Geometry: final body of the model. Coordinates: model frame, mm. Face numbers are marked on the shaded views. Round coordinates to 2 decimals unless told otherwise and drop trailing zeros. Order: outer loops, then holes, each group sorted by start corner. A loop starts at its lowest first (then second) coordinate and runs counter-clockwise, first axis right, second up. Notation, with made-up numbers: (21.5, -37.5) - (80.5, -37.5) arc R26 cw to (80.5, -12.5) - close; hole circle Ø5 at (45.25, 53.25). An arc over 180 degrees is marked (long way). Put each result on its own line as item: value. Start each with the question number.
(1) Material intervals for L1, parallel to X at y = 9.15, z = 0; L2, parallel to X at y = 9.45, z = 18.5; L3, parallel to X at y = 8.7, z = 22, sorted ascending. Write a range as [from, to].
(2) Section C-C (z = 24). Output: boundary loops of the cut face in (x, y).
(3) Pull-direction query (Y, two-part tool) for the marked faces 1 and 2; classes: released by +Y, released by -Y, zero draft, split by the parting line, or undercut.
(4) Section B-B (y = 8.9). Output: boundary loops of the cut face in (x, z).
(5) Section D-D (z = -38). Output: boundary loops of the cut face in (x, y).
(6) Pin query (flat end, axial travel): P1, Ø0.8, axis at x = -1.5, y = 9, coming from the -Z side; P2, Ø1.5, axis at x = -32.91, z = 19, coming from the -Y side. Return the tip coordinate at first contact, or that it passes through.
(7) Section A-A (z = 0). Output: boundary loops of the cut face in (x, y).
from build123d import *

# Parameters (mm, degrees)
SKETCH_1_R      = 1.25
EXTRUDE_1_DEPTH = 1.6
FILLET_1_R      = 3


with BuildPart() as part:
    # 草图1 → 凸台-拉伸1 (new body)
    with BuildSketch(Plane(origin=(0, 8.4, 0), x_dir=(1, 0, 0), z_dir=(0, 1, 0))):
        with BuildLine():
            ThreePointArc((-42.584930161, -28.625185914), (-36.646174274, -35.915671462), (-29.47672888, -42))
            Line((-29.47672888, -42), (29.47672888, -42))
            ThreePointArc((29.47672888, -42), (36.646174274, -35.915671462), (42.584930161, -28.625185914))
            Line((42.584930161, -28.625185914), (39.709874377, -26.965271683))
            ThreePointArc((39.709874377, -26.965271683), (38.538130468, -22.25), (43.207547486, -20.90712415))
            Line((43.207547486, -20.90712415), (46.08260327, -22.567038381))
            ThreePointArc((46.08260327, -22.567038381), (44.43712591, 25.655786606), (3.497673109, 51.192224295))
            Line((3.497673109, 51.192224295), (3.497673109, 47.872395833))
            ThreePointArc((3.497673109, 47.872395833), (0, 44.5), (-3.497673109, 47.872395833))
            Line((-3.497673109, 47.872395833), (-3.497673109, 51.192224295))
            ThreePointArc((-3.497673109, 51.192224295), (-44.43712591, 25.655786606), (-46.08260327, -22.567038381))
            Line((-46.08260327, -22.567038381), (-43.207547486, -20.90712415))
            ThreePointArc((-43.207547486, -20.90712415), (-38.538130468, -22.25), (-39.709874377, -26.965271683))
            Line((-39.709874377, -26.965271683), (-42.584930161, -28.625185914))
        make_face()
        with Locations(Location((-32.908965344, -19, 0), (0, 0, 270))):
            Circle(SKETCH_1_R, mode=Mode.SUBTRACT)
        with Locations(Location((32.908965344, -19, 0), (0, 0, 270))):
            Circle(SKETCH_1_R, mode=Mode.SUBTRACT)
        with BuildLine():
            Line((6.244997998, -19), (-6.244997998, -19))
            ThreePointArc((-6.244997998, -19), (0, 20), (6.244997998, -19))
        make_face(mode=Mode.SUBTRACT)
        with Locations(Location((0, 38, 0), (0, 0, 270))):
            Circle(SKETCH_1_R, mode=Mode.SUBTRACT)
    extrude(amount=EXTRUDE_1_DEPTH)

    # 圆角1
    fillet_1_edges = [part.edges().sort_by_distance(p)[0] for p in [
        (-29.47672888, 9.2, 42),
        (29.47672888, 9.2, 42),
        (-6.244997998, 9.2, 19),
        (6.244997998, 9.2, 19),
    ]]
    fillet(fillet_1_edges, radius=FILLET_1_R)


solid = part.part
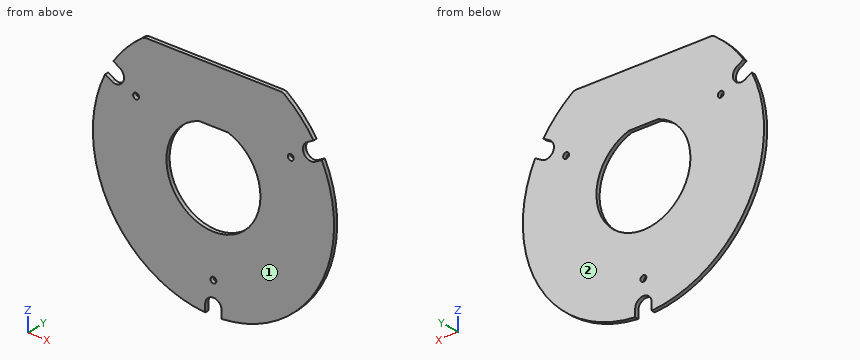
Checks:
1. L1: x = [-51.31, -20], [20, 51.31]
1. L2: x = [-47.86, -34.05], [-31.76, -7.6], [7.6, 31.76], [34.05, 47.86]
1. L3: x = [-46.36, -45.1], [-38.7, 38.7], [45.1, 46.36]
2. outline: (-38.07, 8.4) - (38.07, 8.4) - (38.07, 10) - (-38.07, 10) - close
3. face 1: released by -Y
3. face 2: released by +Y
4. outline: (-46.08, 22.57) arc R51.31 ccw to (-3.5, -51.19) - (-3.5, -47.87) arc R3.5 cw to (3.5, -47.87) - (3.5, -51.19) arc R51.31 ccw to (46.08, 22.57) - (43.21, 20.91) arc R3.5 cw to (39.71, 26.97) - (42.58, 28.63) arc R51.31 ccw to (30.28, 41.42) arc R3 ccw to (28.51, 42) - (-28.51, 42) arc R3 ccw to (-30.28, 41.42) arc R51.31 ccw to (-42.58, 28.63) - (-39.71, 26.97) arc R3.5 cw to (-43.21, 20.91) - close; hole circle Ø2.5 at (-32.91, 19); hole (-6.76, 18.82) arc R20 ccw (long way) to (6.76, 18.82) arc R3 ccw to (5.74, 19) - (-5.74, 19) arc R3 ccw to start; hole circle Ø2.5 at (0, -38); hole circle Ø2.5 at (32.91, 19)
5. outline: (-34.48, 8.4) - (-1.25, 8.4) - (-1.25, 10) - (-34.48, 10) - close; (1.25, 8.4) - (34.48, 8.4) - (34.48, 10) - (1.25, 10) - close
6. P1: stops at z = -45.06
6. P2: passes through
7. outline: (-51.31, 8.4) - (-20, 8.4) - (-20, 10) - (-51.31, 10) - close; (20, 8.4) - (51.31, 8.4) - (51.31, 10) - (20, 10) - close
